Read the model definition and answer for the solid it produces. Units are mm, in the model's axes. Give positions to 0.01 mm unless a question says otherwise; leave off trailing zeros. Order: outer loops, then holes, each group sorted by start corner. A loop starts at its lowest first (then second) coordinate and runs counter-clockwise, first axis right, second up.
Item 1: A cutting plane is placed at A-A (x = 133). Write down the section's boundary in (y, z) (3 decimals), plus the area to 3 significant figures.
Item 2: Find the intervals of material crossed by line 1 along Y through (x, z) = (114, -2.15) (3 decimals); line 2 along Y through (x, z) = (110, -0.55) (3 decimals); line 3 along X through (y, z) = (-95, -1.65), in increasing order.
Item 3: A cutting plane is placed at D-D (y = -138). Write down the section's boundary in (x, z) (3 decimals).
Item 4: Given pin 1 Ø1.6 at (x, z) = (179.5, -1.5) entering from +Y; pin 2 Ø1.6 at (y, z) = (-158, -2.5) entering from -X; pin 3 Ø1 at (x, z) = (83.5, -2) entering from +Y, each flat-ended and moving along its own axis, determine where each tip first touches the part or whether it passes through.
Item 5: A cutting plane is placed at B-B (y = -51). Write down the section's boundary in (x, z) (3 decimals).
Item 6: A cutting plane is placed at C-C (x = -42.5). Write down the section's boundary in (y, z) (3 decimals), plus the area to 3 significant figures.
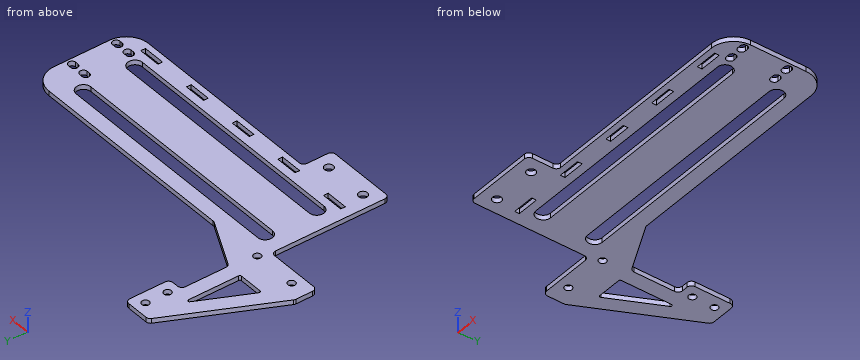
from build123d import *

# Parameters (mm, degrees)
SKETCH1_R           = 3
SKETCH1_R_2         = 2.5
SKETCH1_W           = 15
SKETCH1_H           = 3.175
BASE_FLANGE1_DEPTH  = 3.175
CUT_EXTRUDE1_DEPTH  = 10
SKETCH3_W           = 10
SKETCH3_H           = 30
BOSS_EXTRUDE1_DEPTH = 3.175
FILLET2_R           = 3
FILLET1_R           = 15
FILLET3_R           = 1
SKETCH4_R           = 2.5
CUT_EXTRUDE2_DEPTH  = 10
SKETCH5_W           = 6.305242908
SKETCH5_H           = 6.547752252
BOSS_EXTRUDE2_DEPTH = 3.175


# Sheet-metal steps are written as plain solids
with BuildPart() as part:
    # Sketch1 → Base-Flange1 (new body)
    with BuildSketch(Plane.XY):
        Polygon((-4.193265857, -88), (25.47, -95.5), (185, -95.5), (185, -143.5), (185, -148.5), (185, -163.175), (35, -163.175), (35, -183.175), (-15, -183.175), (-15, -163.175), (-15, -150.03), (-15, -103), (-55, -103), (-55, -88), align=None)
        with Locations((-5, -173.175)):
            Circle(SKETCH1_R, mode=Mode.SUBTRACT)
        with Locations((25, -173.175)):
            Circle(SKETCH1_R, mode=Mode.SUBTRACT)
        with Locations((-42.5, -95.5)):
            Circle(SKETCH1_R_2, mode=Mode.SUBTRACT)
        with Locations((-12.5, -95.5)):
            Circle(SKETCH1_R_2, mode=Mode.SUBTRACT)
        with Locations((160, -157.5875)):
            Rectangle(SKETCH1_W, SKETCH1_H, mode=Mode.SUBTRACT)
        with Locations((40, -157.5875)):
            Rectangle(SKETCH1_W, SKETCH1_H, mode=Mode.SUBTRACT)
        with Locations((0, -157.5875)):
            Rectangle(SKETCH1_W, SKETCH1_H, mode=Mode.SUBTRACT)
        with Locations((80, -157.5875)):
            Rectangle(SKETCH1_W, SKETCH1_H, mode=Mode.SUBTRACT)
        with Locations((120, -157.5875)):
            Rectangle(SKETCH1_W, SKETCH1_H, mode=Mode.SUBTRACT)
        with BuildLine():
            Line((181, -122.25), (179, -122.25))
            ThreePointArc((179, -122.25), (176.5, -119.75), (179, -117.25))
            Line((179, -117.25), (181, -117.25))
            ThreePointArc((181, -117.25), (183.5, -119.75), (181, -122.25))
        make_face(mode=Mode.SUBTRACT)
        with BuildLine():
            Line((171, -122.25), (169, -122.25))
            ThreePointArc((169, -122.25), (166.5, -119.75), (169, -117.25))
            Line((169, -117.25), (171, -117.25))
            ThreePointArc((171, -117.25), (173.5, -119.75), (171, -122.25))
        make_face(mode=Mode.SUBTRACT)
        with BuildLine():
            Line((171, -147.25), (169, -147.25))
            ThreePointArc((169, -147.25), (166.5, -149.75), (169, -152.25))
            Line((169, -152.25), (171, -152.25))
            ThreePointArc((171, -152.25), (173.5, -149.75), (171, -147.25))
        make_face(mode=Mode.SUBTRACT)
        with BuildLine():
            Line((181, -147.25), (179, -147.25))
            ThreePointArc((179, -147.25), (176.5, -149.75), (179, -152.25))
            Line((179, -152.25), (181, -152.25))
            ThreePointArc((181, -152.25), (183.5, -149.75), (181, -147.25))
        make_face(mode=Mode.SUBTRACT)
    extrude(amount=-BASE_FLANGE1_DEPTH)

    # Sketch2 → Cut-Extrude1 (cut)
    with BuildSketch(Plane.XY):
        with BuildLine():
            Line((0, -105.5), (159, -105.5))
            ThreePointArc((159, -105.5), (164, -110.5), (159, -115.5))
            Line((159, -115.5), (0, -115.5))
            ThreePointArc((0, -115.5), (-5, -110.5), (0, -105.5))
        make_face()
        with BuildLine():
            Line((0, -140.5), (159, -140.5))
            ThreePointArc((159, -140.5), (164, -145.5), (159, -150.5))
            Line((159, -150.5), (0, -150.5))
            ThreePointArc((0, -150.5), (-5, -145.5), (0, -140.5))
        make_face()
    extrude(amount=-CUT_EXTRUDE1_DEPTH, mode=Mode.SUBTRACT)

    # Sketch3 → Boss-Extrude1 (add)
    # profile 1 of 3: a face of its own
    with BuildSketch(Plane.XY):
        Polygon((-20, -15.5), (-55, -88), (-10, -88), (-10, -78), (-10, -45.5), (-10, -15.5), align=None)
        Polygon((-20, -38.501774554), (-20, -78), (-39.068108836, -78), align=None, mode=Mode.SUBTRACT)
    # profile 2 of 3: a face of its own
    with BuildSketch(Plane.XY):
        Polygon((-10, -78), (-10, -88), (25.47, -95.5), align=None)
    # profile 3 of 3: a face of its own
    with BuildSketch(Plane.XY):
        with Locations((-5, -30.5)):
            Rectangle(SKETCH3_W, SKETCH3_H)
    extrude(amount=-BOSS_EXTRUDE1_DEPTH)

    # Fillet2
    fillet2_edges = [part.edges().sort_by_distance(p)[0] for p in [
        (25.47, -95.5, -1.5875),
        (35, -163.175, -1.5875),
        (35, -183.175, -1.5875),
        (-15, -183.175, -1.5875),
        (-15, -103, -1.5875),
        (-55, -103, -1.5875),
        (-55, -88, -1.5875),
        (0, -45.5, -1.5875),
        (0, -15.5, -1.5875),
        (-20, -15.5, -1.5875),
        (-10, -78, -1.5875),
        (-10, -45.5, -1.5875),
    ]]
    fillet(fillet2_edges, radius=FILLET2_R)

    # Fillet1
    fillet1_edges = [part.edges().sort_by_distance(p)[0] for p in [
        (185, -95.5, -1.5875),
        (185, -163.175, -1.5875),
    ]]
    fillet(fillet1_edges, radius=FILLET1_R)

    # Fillet3
    fillet3_edges = [part.edges().sort_by_distance(p)[0] for p in [
        (-20, -78, -1.5875),
        (-39.068108836, -78, -1.5875),
        (-20, -38.501774554, -1.5875),
    ]]
    fillet(fillet3_edges, radius=FILLET3_R)

    # Sketch4 → Cut-Extrude2 (cut)
    with BuildSketch(Plane.XY):
        with Locations((-8, -23)):
            Circle(SKETCH4_R)
        with Locations((-8, -38)):
            Circle(SKETCH4_R)
    extrude(amount=-CUT_EXTRUDE2_DEPTH, mode=Mode.SUBTRACT)

    # Sketch5 → Boss-Extrude2 (add)
    with BuildSketch(Plane.XY):
        with Locations((-8.695694073, -86.656931436)):
            Rectangle(SKETCH5_W, SKETCH5_H)
    extrude(amount=-BOSS_EXTRUDE2_DEPTH)


solid = part.part
Response values:
1. outline: (-163.175, -3.175) - (-150.5, -3.175) - (-150.5, 0) - (-163.175, 0) - close; (-140.5, -3.175) - (-115.5, -3.175) - (-115.5, 0) - (-140.5, 0) - close; (-105.5, -3.175) - (-95.5, -3.175) - (-95.5, 0) - (-105.5, 0) - close
1. area: 151 mm2
2. line 1: y = -163.175 to -159.175, -156 to -150.5, -140.5 to -115.5, -105.5 to -95.5
2. line 2: y = -163.175 to -150.5, -140.5 to -115.5, -105.5 to -95.5
2. line 3: x = -55 to -44.95, -40.05 to -14.95, -10.05 to 24.46
3. outline: (-15, -3.175) - (185, -3.175) - (185, 0) - (-15, 0) - close
4. pin 1: stops at y = -98.28
4. pin 2: stops at x = -15
4. pin 3: stops at y = -95.5
5. outline: (-37.138, -3.175) - (-26.034, -3.175) - (-26.034, 0) - (-37.138, 0) - close; (-20, -3.175) - (-10, -3.175) - (-10, 0) - (-20, 0) - close
6. outline: (-103, -3.175) - (-98, -3.175) - (-98, 0) - (-103, 0) - close; (-93, -3.175) - (-62.107, -3.175) - (-62.107, 0) - (-93, 0) - close
6. area: 114 mm2
